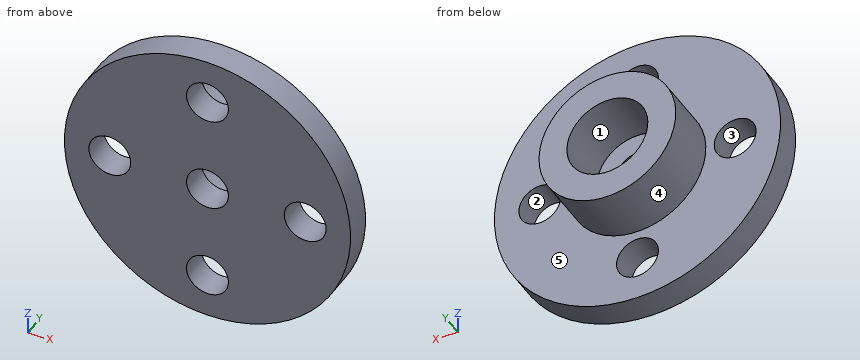
from build123d import *

# Parameters (mm, degrees)
SKETCH1_R           = 10.25
BOSS_EXTRUDE1_DEPTH = 2
SKETCH2_R           = 1.5
CUT_EXTRUDE1_DEPTH  = 3
SKETCH3_R           = 4.9
SKETCH3_R_2         = 2.9
BOSS_EXTRUDE2_DEPTH = 4


with BuildPart() as part:
    # Sketch1 → Boss-Extrude1 (new body)
    with BuildSketch(Plane(origin=(0, 0, 0), x_dir=(1, 0, 0), z_dir=(0, 1, 0))):
        with Locations(Location((0, 0, 0), (0, 0, 270))):
            Circle(SKETCH1_R)
    extrude(amount=BOSS_EXTRUDE1_DEPTH)

    # Sketch2 → Cut-Extrude1 (cut)
    with BuildSketch(Plane(origin=(0, 2, 0), x_dir=(1, 0, 0), z_dir=(0, 1, 0))):
        with Locations(Location((7, 0, 0), (0, 0, 270))):
            Circle(SKETCH2_R)
        with Locations(Location((0, 0, 0), (0, 0, 270))):
            Circle(SKETCH2_R)
        with Locations(Location((0, 7, 0), (0, 0, 270))):
            Circle(SKETCH2_R)
        with Locations(Location((-7, 0, 0), (0, 0, 270))):
            Circle(SKETCH2_R)
        with Locations(Location((0, -7, 0), (0, 0, 270))):
            Circle(SKETCH2_R)
    extrude(amount=-CUT_EXTRUDE1_DEPTH, mode=Mode.SUBTRACT)

    # Sketch3 → Boss-Extrude2 (add)
    with BuildSketch(Plane(origin=(0, 2, 0), x_dir=(1, 0, 0), z_dir=(0, 1, 0))):
        with Locations(Location((0, 0, 0), (0, 0, 270))):
            Circle(SKETCH3_R)
        with Locations(Location((0, 0, 0), (0, 0, 270))):
            Circle(SKETCH3_R_2, mode=Mode.SUBTRACT)
    extrude(amount=BOSS_EXTRUDE2_DEPTH)


solid = part.part
Design review of the part built by this model. Coordinates are the model's own, in mm. Face numbers are marked on the shaded views. A direction names the side the tool comes from. Give positions to 0.01 mm unless a question says otherwise; leave off trailing zeros. Loops run counter-clockwise (first coordinate to the right, second up) from the corner with the lowest first, then second, coordinate; pieces in that order, holes last. Notation, with made-up numbers: (52, 18) - (95, 18) arc R24 ccw to (95, 39) - close; hole circle Ø1 at (29, 64). An arc over 180 degrees is marked (long way). Write item = value, one per line.
1) Take a section at A-A on x = 0. State the section outline as (y, z) points.
Result sheet:
outline = (0, -10.25) - (2, -10.25) - (2, -8.5) - (0, -8.5) - close; (0, -5.5) - (2, -5.5) - (2, -4.9) - (6, -4.9) - (6, -2.9) - (2, -2.9) - (2, -1.5) - (0, -1.5) - close; (0, 1.5) - (2, 1.5) - (2, 2.9) - (6, 2.9) - (6, 4.9) - (2, 4.9) - (2, 5.5) - (0, 5.5) - close; (0, 8.5) - (2, 8.5) - (2, 10.25) - (0, 10.25) - close
2) To check wall thickness, follow line 1 (X direction, y = 1.5, z = 0); line 2 (X direction, y = 3.2, z = 0); line 3 (Y direction, x = -3.75, z = -5.25). State the ranges of each line that lie inside material, in increasing order.
Result sheet:
line_1 = -10.25 to -8.5, -5.5 to -1.5, 1.5 to 5.5, 8.5 to 10.25
line_2 = -4.9 to -2.9, 2.9 to 4.9
line_3 = 0 to 2
3) Take a section at C-C on x = 7. State the section outline as (y, z) points, and give its area (4 significant figures).
Result sheet:
outline = (0, -7.49) - (2, -7.49) - (2, -1.5) - (0, -1.5) - close; (0, 1.5) - (2, 1.5) - (2, 7.49) - (0, 7.49) - close
area = 23.95 mm2
4) Take a section at B-B on z = 6.75. State the section outline as (x, y) points.
Result sheet:
outline = (-7.71, 0) - (-1.48, 0) - (-1.48, 2) - (-7.71, 2) - close; (1.48, 0) - (7.71, 0) - (7.71, 2) - (1.48, 2) - close
5) Take a section at D-D on z = -1. State the section outline as (x, y) points.
Result sheet:
outline = (-10.2, 0) - (-8.12, 0) - (-8.12, 2) - (-10.2, 2) - close; (-5.88, 0) - (-1.12, 0) - (-1.12, 2) - (-2.72, 2) - (-2.72, 6) - (-4.8, 6) - (-4.8, 2) - (-5.88, 2) - close; (1.12, 0) - (5.88, 0) - (5.88, 2) - (4.8, 2) - (4.8, 6) - (2.72, 6) - (2.72, 2) - (1.12, 2) - close; (8.12, 0) - (10.2, 0) - (10.2, 2) - (8.12, 2) - close
6) Draft analysis for pull direction Z (two halves, no side actions). For the marked faces 3, 4 and 5, state which applies: +Z half, -Z half, draft (parallel to the pull), parting line (faces both ways), or undercut.
Result sheet:
face_3 = undercut
face_4 = parting line
face_5 = draft
7) Tool access review of the marked faces 1 and 2: name each direction out of +Z, -Z, +X, -X, +Y, -Y from which nothing blocks a thin tool from reaching the whole face with its end or side.
Result sheet:
face_1 = +Y
face_2 = +Y, -Y
8) Clearance check with flat-ended pins moving along their axes: pin 1 Ø1 at (x, z) = (8, -4.5) entering from +Y; pin 2 Ø1.5 at (x, y) = (-1.5, 2.5) entering from +Z. State where each tip first meets the part, or that it passes through.
Result sheet:
pin_1 = 2
pin_2 = 10.21
